```python
from build123d import *

# Parameters (mm, degrees)
F0_W = 4.500004
F0_H = 15


with BuildPart() as f2:
    # F0 (on Front) → F2 (revolve)
    with BuildSketch(Plane.XZ):
        Polygon((6.250002, 5), (6.250002, 8), (2.250002, 8), (-2.250002, 8), (-6.250002, 8), (-6.250002, 5), align=None)
        with Locations((0, 15.5)):
            Rectangle(F0_W, F0_H)
        with BuildLine():
            Line((-2.250002, 23), (2.250002, 23))
            ThreePointArc((2.250002, 23), (0, 42.743587), (-2.250002, 23))
        make_face()
    revolve(axis=Axis((9.867935, 0, 0), (1, 0, 0)))


solid = f2.part
```
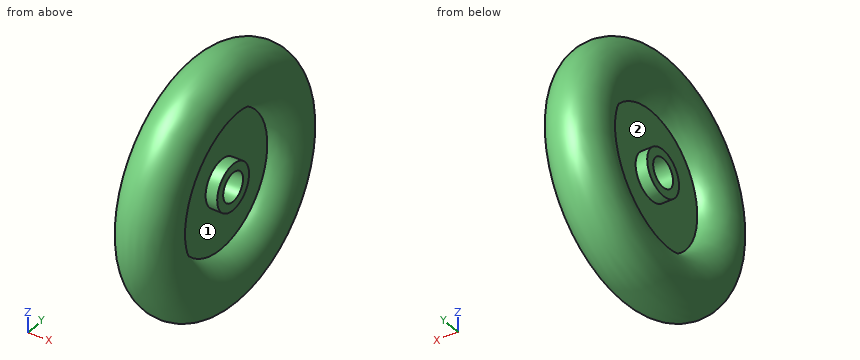
Verification items for the finished model (mm, model axes). Face numbers are marked on the shaded views. Round coordinates to 2 decimals unless told otherwise and drop trailing zeros. Order: outer loops, then holes, each group sorted by start corner. A loop starts at its lowest first (then second) coordinate and runs counter-clockwise, first axis right, second up.
1) Depth check by flat-ended pin: pin 1 (8 mm diameter, centred on y = 23.5, z = -9.5, fed in from -X); pin 2 (8 mm diameter, centred on y = -2.5, z = 3.5, fed in from -X); pin 3 (4 mm diameter, centred on y = -16.5, z = 4, fed in from +X). Enter the tip coordinate at first touch or a pass-through.
Geometry says:
pin 1: stops at x = -9.41
pin 2: stops at x = -6.25
pin 3: stops at x = 2.25
2) Material ranges on line 1 (Z direction, x = 2.5, y = 0); line 2 (Z direction, x = 3, y = 0), recorded low to high.
Geometry says:
line 1: z = -42.43 to -23.06, -8 to -5, 5 to 8, 23.06 to 42.43
line 2: z = -42.28 to -23.2, -8 to -5, 5 to 8, 23.2 to 42.28
3) Cross-section at C-C, the plane x = -1.25. Record the cut outline in (y, z), plus the area to 3 significant figures.
Geometry says:
outline: circle Ø85.33 at (0, 0); hole circle Ø10 at (0, 0)
area: 5,640 mm2
4) Cross-section at A-A, the plane y = 0. Record the cut outline in (x, z).
Geometry says:
outline: (-6.25, -8) - (-2.25, -8) - (-2.25, -23) arc R10 ccw (long way) to (2.25, -23) - (2.25, -8) - (6.25, -8) - (6.25, -5) - (-6.25, -5) - close; (-6.25, 5) - (6.25, 5) - (6.25, 8) - (2.25, 8) - (2.25, 23) arc R10 ccw (long way) to (-2.25, 23) - (-2.25, 8) - (-6.25, 8) - close
5) Draft check along Z on the marked faces 1 and 2. Enter one of: +Z half, -Z half, draft (parallel to the pull), parting line (faces both ways), or undercut.
Geometry says:
face 1: undercut
face 2: undercut
